The drawing under review shows one solid part. Ordinate dimensions are in mm from its lowest x, y, z. A direction names the side the tool comes from. Round coordinates to 2 decimals unless told otherwise and drop trailing zeros. Loops run counter-clockwise (first coordinate to the right, second up) from the corner with the lowest first, then second, coordinate; pieces in that order, holes last. Notation, with made-up numbers: (84, 25) -> (139, 25) arc R15 ccw to (139, 35) -> close; hole circle Ø9 at (-20.5, -36.75). An arc over 180 degrees is marked (long way). Use a Markdown table: item, result. Add a question column.
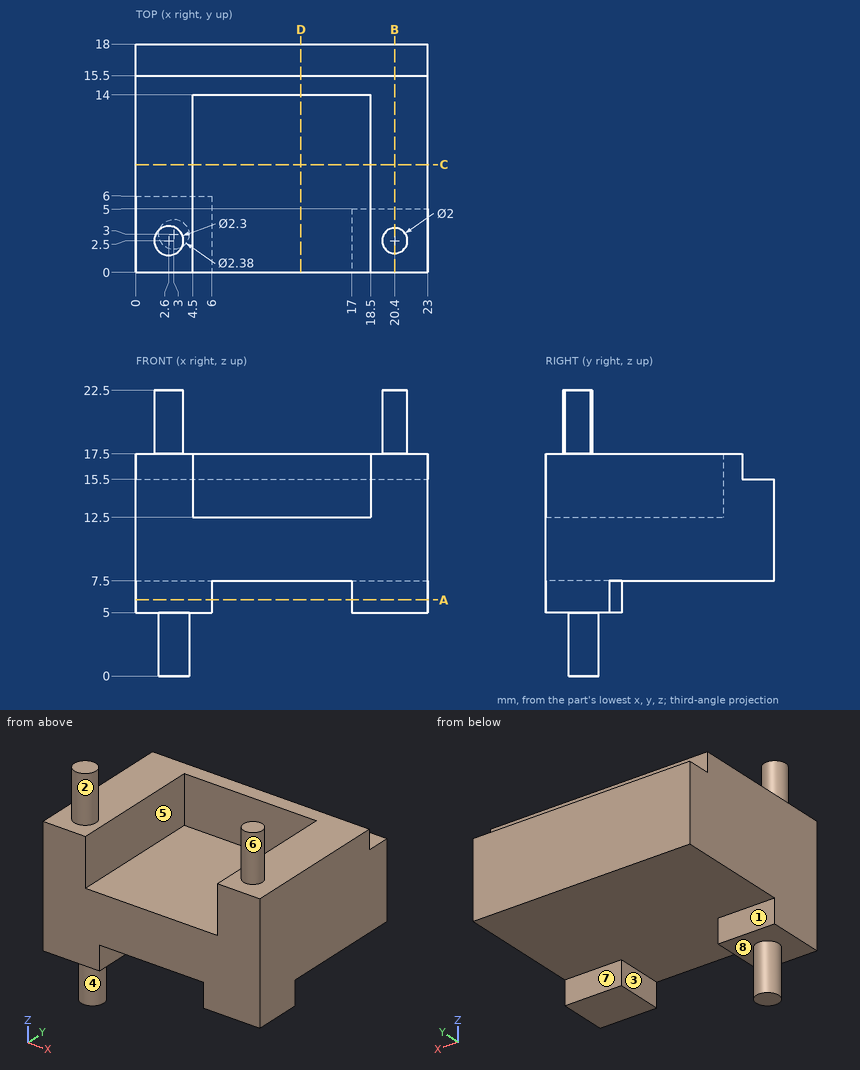
1. Consider section B-B on x = 20.4. State the section outline as (y, z) points.
2. Mouldability with a two-part tool opening along X and no side actions: class the marked faces 1, 2, 3 and 4 as +X half, -X half, draft (parallel to the pull), parting line (faces both ways), or undercut.
3. Consider section C-C on y = 8.5. State the section outline as (x, z) points.
4. Consider section D-D on x = 13. State the section outline as (y, z) points, plus the area to 3 significant figures.
5. Consider section A-A on z = 6. State the section outline as (x, y) points.
6. To check wall thickness, follow probe 1 along X at (y, z) = (3.5, 14.75); probe 2 along Z at (x, y) = (15, 7); probe 3 along Y at (x, z) = (5.25, 13). State the ranges of each line that lie inside material, in increasing order. Write a range as from..to.
7. Insertion check: P1, Ø4, axis at x = 13, z = 15.5, coming from the -Y side; P2, Ø3, axis at x = 15.5, y = 17.5, coming from the +Z side; P3, Ø6.5, axis at x = 2.5, y = 2.5, coming from the -Z side; P4, Ø1.5, axis at x = 9, z = 6, coming from the -Y side. Each pin has a flat end and moves straight along its axis. Give the tip position at first contact, or say it passes through.
8. For the marked faces 5, 6, 7 and 8, list the 3-axis set-ups (+Z, -Z, +X, -X, +Y, -Y) from which the entire face can be reached by the end or side of a thin tool; tool diameter is ignored.
Verdict:
| question | item | result |
|---|---|---|
| 1 | outline | (0, 5) -> (5, 5) -> (5, 7.5) -> (18, 7.5) -> (18, 15.5) -> (15.5, 15.5) -> (15.5, 17.5) -> (3.5, 17.5) -> (3.5, 22.5) -> (1.5, 22.5) -> (1.5, 17.5) -> (0, 17.5) -> close |
| 2 | face 1 | draft |
| 2 | face 2 | undercut |
| 2 | face 3 | undercut |
| 2 | face 4 | parting line |
| 3 | outline | (0, 7.5) -> (23, 7.5) -> (23, 17.5) -> (18.5, 17.5) -> (18.5, 12.5) -> (4.5, 12.5) -> (4.5, 17.5) -> (0, 17.5) -> close |
| 4 | outline | (0, 7.5) -> (18, 7.5) -> (18, 15.5) -> (15.5, 15.5) -> (15.5, 17.5) -> (14, 17.5) -> (14, 12.5) -> (0, 12.5) -> close |
| 4 | area | 105 mm² |
| 5 | outline | (0, 0) -> (6, 0) -> (6, 6) -> (0, 6) -> close; (17, 0) -> (23, 0) -> (23, 5) -> (17, 5) -> close |
| 6 | probe 1 | x = 0..4.5, 18.5..23 |
| 6 | probe 2 | z = 7.5..12.5 |
| 6 | probe 3 | y = 14..18 |
| 7 | P1 | stops at y = 14 |
| 7 | P2 | stops at z = 15.5 |
| 7 | P3 | stops at z = 0 |
| 7 | P4 | passes through |
| 8 | face 5 | +Z, -Y |
| 8 | face 6 | +Z |
| 8 | face 7 | -Z, +X, +Y |
| 8 | face 8 | -Z |
